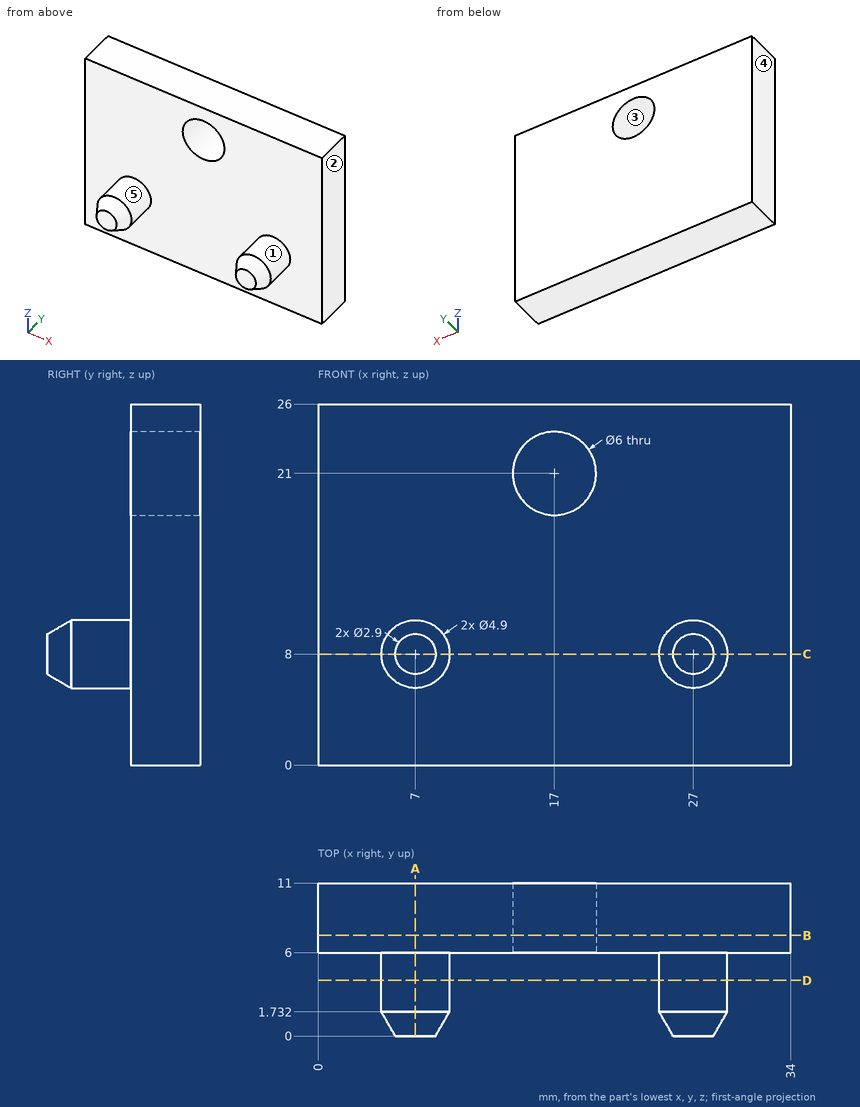
For this review, use the dimensioned drawing (mm, ordinates from the lowest corner) and the shaded views. A direction names the side the tool comes from. Give positions to 0.01 mm unless a question says otherwise; leave off trailing zeros. Write each loop counter-clockwise with the first axis right and the second up, starting at its lowest first coordinate (ties: lowest second). Pieces come first, ordered by that corner, then holes. Notation, with made-up numbers: M -21.5,-2 L 5.5,-2 A28 cw 5.5,22 Z; hole C -29.5,66 d3. An arc over 180 degrees is marked long. Write item = value, one per line. Start each with the question number.
Q1. Machinability: for the marked faces 4 and 5, which of the approach directions +Z, -Z, +X, -X, +Y, -Y give a long, thin tool a straight path to every point of the face, cutting with its end or side? Answer none if there is none.
Q2. Mouldability with a two-part tool opening along Z and no side actions: class the marked faces 1, 2 and 3 as released by +Z, released by -Z, zero draft, split by the parting line, or undercut.
Q3. For line 1 (X direction, y = 3, z = 8); line 2 (X direction, y = 9.25, z = 21); line 3 (Y direction, x = 23.5, z = 21.25), list the stretches that pass through material, from the lowest coordinate up.
Q4. Clearance check with flat-ended pins moving along their axes: pin 1 (1 mm diameter, centred on x = 12.5, z = 17, fed in from -Y); pin 2 (10 mm diameter, centred on x = 24, z = 14, fed in from -Y). State where each tip first meets the part, or that it passes through.
Q5. We need section B-B (y = 7.25). State the section outline as (x, z) points, plus the area to 3 significant figures.
Q6. We need section D-D (y = 4). State the section outline as (x, z) points, plus the area to 3 significant figures.
Q7. We need section C-C (z = 8). State the section outline as (x, y) points.
Q8. We need section A-A (x = 7). State the section outline as (y, z) points.
Result set:
q1.face_4 = +Z, -Z, -X, +Y, -Y
q1.face_5 = -Y
q2.face_1 = split by the parting line
q2.face_2 = zero draft
q2.face_3 = undercut
q3.line_1 = 4.55 to 9.45, 24.55 to 29.45
q3.line_2 = 0 to 14, 20 to 34
q3.line_3 = 6 to 11
q4.pin_1 = 6
q4.pin_2 = 0.45
q5.outline = M 0,0 L 34,0 L 34,26 L 0,26 Z; hole C 17,21 d6
q5.area = 856 mm2
q6.outline = C 7,8 d4.9; C 27,8 d4.9
q6.area = 37.7 mm2
q7.outline = M 0,6 L 4.55,6 L 4.55,1.73 L 5.55,0 L 8.45,0 L 9.45,1.73 L 9.45,6 L 24.55,6 L 24.55,1.73 L 25.55,0 L 28.45,0 L 29.45,1.73 L 29.45,6 L 34,6 L 34,11 L 0,11 Z
q8.outline = M 0,6.55 L 1.73,5.55 L 6,5.55 L 6,0 L 11,0 L 11,26 L 6,26 L 6,10.45 L 1.73,10.45 L 0,9.45 Z
